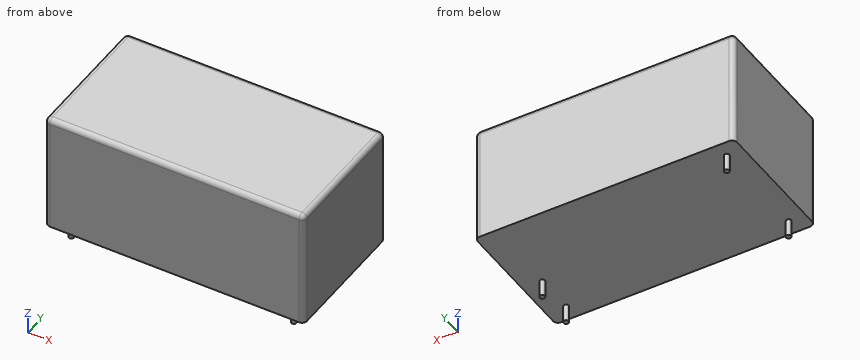
```python
from build123d import *

# Parameters (mm, degrees)
F0_W     = 52.4
F0_H     = 27.2
F1_DEPTH = 24
F2_R     = 0.52
F3_DEPTH = 3.5
F4_R     = 1


with BuildPart() as f1:
    # F0 (on Top) → F1 (new body)
    with BuildSketch(Plane.XY):
        with Locations((26.2, 13.6)):
            Rectangle(F0_W, F0_H)
    extrude(amount=F1_DEPTH)

    # F2 (on Top) → F3 (join)
    with BuildSketch(Plane.XY):
        with Locations((3.4, 3.2)):
            Circle(F2_R)
        with Locations((3.4, 24)):
            Circle(F2_R)
        with Locations((48.4, 3.2)):
            Circle(F2_R)
        with Locations((48.4, 11.2)):
            Circle(F2_R)
    extrude(amount=-F3_DEPTH)

    # F4
    f4_edges = [f1.edges().sort_by_distance(p)[0] for p in [
        (0, 0, 12),
        (52.4, 0, 12),
        (0, 27.2, 12),
        (0, 13.6, 24),
        (26.2, 27.2, 24),
        (52.4, 27.2, 12),
        (52.4, 13.6, 24),
        (26.2, 0, 24),
    ]]
    fillet(f4_edges, radius=F4_R)


solid = f1.part
```
Input: part model. Units: mm. Frame: model coordinates. Coordinates: 2 decimals unless noted, no trailing zeros. Write each loop counter-clockwise with the first axis right and the second up, starting at its lowest first coordinate (ties: lowest second). Pieces come first, ordered by that corner, then holes. Notation, with made-up numbers: (81.5, 47) -> (116.5, 47) arc R26 ccw to (116.5, 80) -> close; hole circle Ø2 at (-38, -14.5). An arc over 180 degrees is marked (long way). Answer as a JSON object with one key per item and string values.
1. Material intervals for line 1 (Z direction, x = 37.5, y = 24), sorted ascending. Write a range as from..to.
Result set:
{"line 1": "z = 0..24"}
2. First-contact query: P1, Ø1, axis at x = 22, y = 22.5, coming from the -Z side. Flat tip, straight axial feed; report the tip coordinate or a pass-through.
Result set:
{"P1": "stops at z = 0"}
3. Section A-A on y = 21.75. Return the cut outline in (x, z), then the cut area to 3 significant figures.
Result set:
{"outline": "(0, 0) -> (52.4, 0) -> (52.4, 23) arc R1 ccw to (51.4, 24) -> (1, 24) arc R1 ccw to (0, 23) -> close", "area": "1,260 mm2"}
4. Section B-B on x = 4.5. Return the cut outline in (y, z), then the cut area to 3 significant figures.
Result set:
{"outline": "(0, 0) -> (27.2, 0) -> (27.2, 23) arc R1 ccw to (26.2, 24) -> (1, 24) arc R1 ccw to (0, 23) -> close", "area": "652 mm2"}
